Could you check a few things on this drawing? It's one solid part, dimensions in mm from its lowest x, y, z. Give positions to 0.01 mm unless a question says otherwise; leave off trailing zeros. Write each loop counter-clockwise with the first axis right and the second up, starting at its lowest first coordinate (ties: lowest second). Pieces come first, ordered by that corner, then holes. Notation, with made-up numbers: (77, 4) -> (132, 4) arc R5 cw to (132, 12) -> close; hole circle Ø4 at (-13.75, 75.25). An arc over 180 degrees is marked (long way). Use CSV: the item, a comma, the result in double quotes. Start each with the question number.
(1) I need wall thicknesses on L1, parallel to Y at x = 6, z = 2.5; L2, parallel to Y at x = 5, z = 1; L3, parallel to Y at x = 6.75, z = 3.25. Which ranges of each line are inside material? Lowest first, please. Write a range as [from, to].
(2) Suppose I cut it at A-A on z = 2.5. List the corners of the cut face in (x, y) for me.
(3) For pin 1 Ø2 at (x, z) = (2, 1) entering from +Y; pin 2 Ø3 at (y, z) = (2.5, 2.5) entering from +X, each with a flat end and sliding along its axis, tell me the tip position at first contact or that it passes through.
(4) If we mould it in two halves opening along Z, with no side actions, what happens to the marked faces 1, 2 and 3? For each: pulls with the +Z half, pulls with the -Z half, needs draft (parallel to the pull), parting line crosses it, or undercut.
(5) Suppose I cut it at C-C on x = 9. List the corners of the cut face in (y, z) for me, plus the area to 3 significant figures.
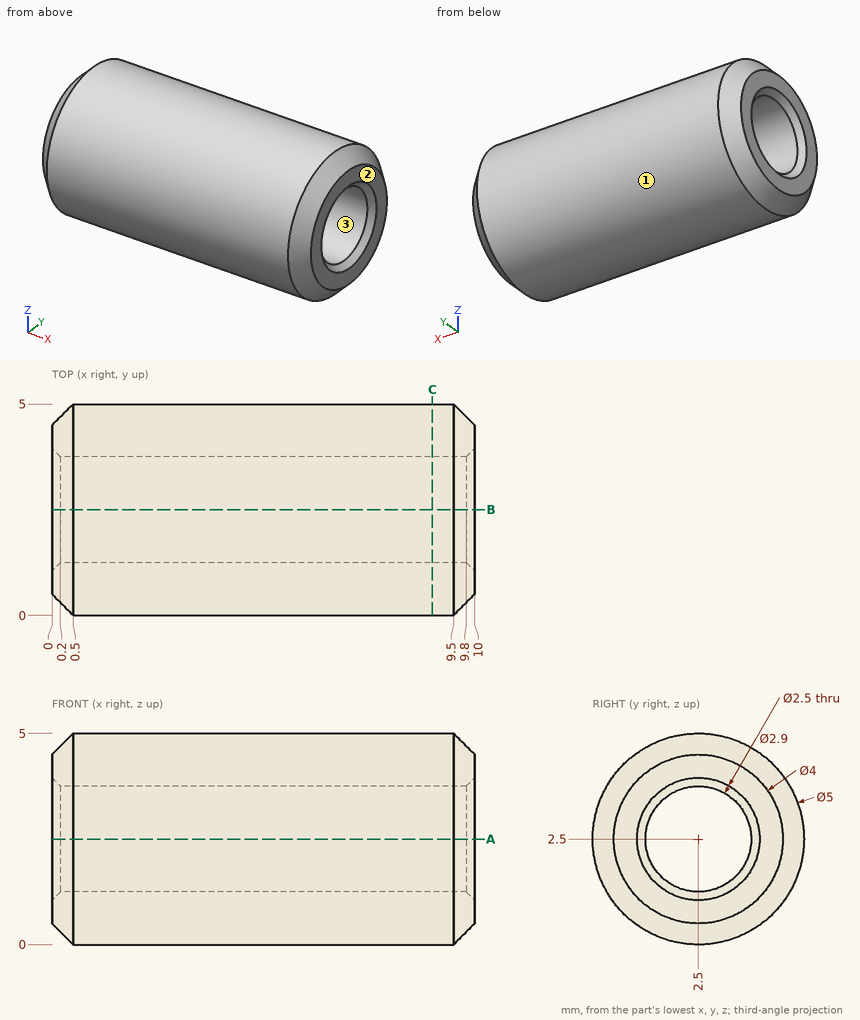
Geometry says:
1,L1,"[0, 1.25], [3.75, 5]"
1,L2,"[0.5, 4.5]"
1,L3,"[0.12, 1.5], [3.5, 4.88]"
2,outline,"(0, 0.5) -> (0.5, 0) -> (9.5, 0) -> (10, 0.5) -> (10, 1.05) -> (9.8, 1.25) -> (0.2, 1.25) -> (0, 1.05) -> close; (0, 3.95) -> (0.2, 3.75) -> (9.8, 3.75) -> (10, 3.95) -> (10, 4.5) -> (9.5, 5) -> (0.5, 5) -> (0, 4.5) -> close"
3,pin 1,"y = 4.95"
3,pin 2,"x = 10"
4,face 1,"parting line crosses it"
4,face 2,"needs draft"
4,face 3,"undercut"
5,outline,"circle Ø5 at (2.5, 2.5); hole circle Ø2.5 at (2.5, 2.5)"
5,area,"14.7 mm²"
